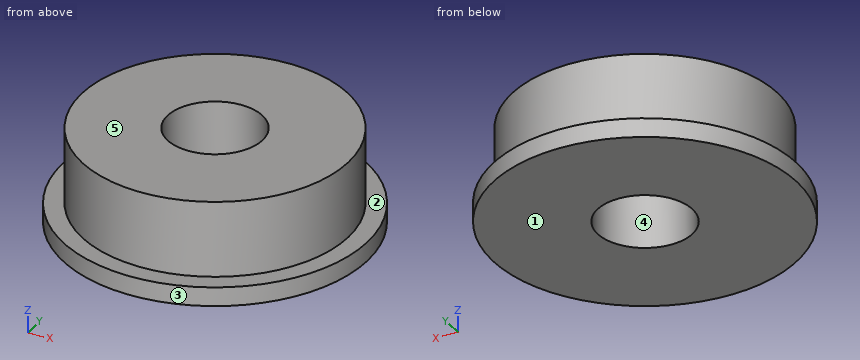
Autodesk Inventor part; units mm, degrees
ref_plane "YZ Plane" through (0, 0, 0) normal (1, 0, 0) x (0, 1, 0)
ref_plane "XZ Plane" through (0, 0, 0) normal (0, 1, 0) x (-1, 0, 0)
ref_plane "XY Plane" through (0, 0, 0) normal (0, 0, 1) x (1, 0, 0)
sketch "Sketch1" plane through (0, 0, 0) normal (0, 0, 1) x (1, 0, 0)
  circle A0 centre (0, 0) radius 8
  dimension "d0" = 16
extrude "Extrusion1" add sketch "Sketch1" along normal blind 1
sketch "Sketch2" plane through (0, 0, 1) normal (0, 0, 1) x (1, 0, 0)
  circle A0 centre (0, 0) radius 8
  circle A1 centre (0, 0) radius 7
  dimension "d4" = 14
extrude "Extrusion2" add sketch "Sketch2" along normal blind 4 contours A1
sketch "Sketch3" plane through (0, 0, 5) normal (0, 0, 1) x (1, 0, 0)
  circle A0 centre (0, 0) radius 7
  circle A1 centre (0, 0) radius 2.5
  dimension "d8" = 5
extrude "Extrusion3" cut sketch "Sketch3" against normal through all contours A1
properties part number "f605zz"
Here's how the part is built. I have some questions about the finished solid (model axes, mm). Face numbers are marked on the shaded views. A direction names the side the tool comes from. Give positions to 0.01 mm unless a question says otherwise; leave off trailing zeros. Order: outer loops, then holes, each group sorted by start corner. A loop starts at its lowest first (then second) coordinate and runs counter-clockwise, first axis right, second up. Notation, with made-up numbers: (35.5, -23.75) - (60.5, -23.75) arc R34 ccw to (60.5, 11.25) - close; hole circle Ø7 at (-22, 41). An arc over 180 degrees is marked (long way). Answer as a JSON object with one key per item and string values. Group by question number.
Item 1: If we mould it in two halves opening along X, with no side actions, what happens to the marked faces 3, 4 and 5? For each: pulls with the +X half, pulls with the -X half, needs draft (parallel to the pull), parting line crosses it, or undercut.
Item 2: Please list where these lines run through material, in increasing order: probe 1 along Y at (x, z) = (0, 3.75); probe 2 along Z at (x, y) = (-4.5, -6.5); probe 3 along X at (y, z) = (-2, 1.85).
Item 3: Which directions (+Z, -Z, +X, -X, +Y, -Y) give clear straight access to the entire face, cutting with the end or side of a thin tool? Please do the marked faces 1 and 2.
Item 4: If we section it at C-C on z = 3.6: Please give me the cut outline in (x, y), and give its area (3 significant figures).
Item 5: If we section it at B-B on x = 2.25: Please give me the cut outline in (y, z).
Item 6: If we section it at A-A on y = 0: Please give me the cut outline in (x, z).
Item 7: For P1, Ø1.5, axis at x = 3, z = 1.5, coming from the +Y side; P2, Ø3, axis at x = 1, z = 3.5, coming from the +Y side, each with a flat end and sliding along its axis, tell me the tip position at first contact or that it passes through.
Item 8: If we section it at D-D on y = -5.75: Please give me the cut outline in (x, z).
Result set:
{
 "1": {"face 3": "parting line crosses it", "face 4": "undercut", "face 5": "needs draft"},
 "2": {"probe 1": "-7 to -2.5, 2.5 to 7", "probe 2": "0 to 1", "probe 3": "-6.71 to -1.5, 1.5 to 6.71"},
 "3": {"face 1": "-Z, +X, -X, +Y, -Y", "face 2": "+Z"},
 "4": {"outline": "circle Ø14 at (0, 0); hole circle Ø5 at (0, 0)", "area": "134 mm²"},
 "5": {"outline": "(-7.68, 0) - (-1.09, 0) - (-1.09, 5) - (-6.63, 5) - (-6.63, 1) - (-7.68, 1) - close; (1.09, 0) - (7.68, 0) - (7.68, 1) - (6.63, 1) - (6.63, 5) - (1.09, 5) - close"},
 "6": {"outline": "(-8, 0) - (-2.5, 0) - (-2.5, 5) - (-7, 5) - (-7, 1) - (-8, 1) - close; (2.5, 0) - (8, 0) - (8, 1) - (7, 1) - (7, 5) - (2.5, 5) - close"},
 "7": {"P1": "y = 7.62", "P2": "y = 7"},
 "8": {"outline": "(-5.56, 0) - (5.56, 0) - (5.56, 1) - (3.99, 1) - (3.99, 5) - (-3.99, 5) - (-3.99, 1) - (-5.56, 1) - close"}
}
